```python
from build123d import *

# Parameters (mm, degrees)
F1_DEPTH = 6.35
F2_R     = 10.668
F3_DEPTH = 2.54
F4_DEPTH = 0.254
F6_SIZE2 = 7.62
F6_SIZE  = 1.524
F7_R     = 1.27


with BuildPart() as f1:
    # F0 (on Top) → F1 (new body)
    with BuildSketch(Plane.XY):
        with BuildLine():
            Line((6.711802813, 0.508), (7.7303263191, 0.508))
            ThreePointArc((7.7303263191, 0.508), (5.4779562339, 5.4779562339), (0.508, 7.7303263191))
            Line((0.508, 7.7303263191), (0.508, 6.711802813))
            ThreePointArc((0.508, 6.711802813), (4.7595357442, 4.7595357442), (6.711802813, 0.508))
        make_face()
    extrude(amount=F1_DEPTH)


with BuildPart() as f1b:
    # F0 (on Top) → F1, piece 2 (new body)
    with BuildSketch(Plane.XY):
        with BuildLine():
            ThreePointArc((-0.508, 7.7303263191), (-5.4779562339, 5.4779562339), (-7.7303263191, 0.508))
            Line((-7.7303263191, 0.508), (-6.711802813, 0.508))
            ThreePointArc((-6.711802813, 0.508), (-4.7595357442, 4.7595357442), (-0.508, 6.711802813))
            Line((-0.508, 6.711802813), (-0.508, 7.7303263191))
        make_face()
    extrude(amount=F1_DEPTH)


with BuildPart() as f1c:
    # F0 (on Top) → F1, piece 3 (new body)
    with BuildSketch(Plane.XY):
        with BuildLine():
            Line((-6.711802813, -0.508), (-7.7303263191, -0.508))
            ThreePointArc((-7.7303263191, -0.508), (-5.4779562339, -5.4779562339), (-0.508, -7.7303263191))
            Line((-0.508, -7.7303263191), (-0.508, -6.711802813))
            ThreePointArc((-0.508, -6.711802813), (-4.7595357442, -4.7595357442), (-6.711802813, -0.508))
        make_face()
    extrude(amount=F1_DEPTH)


with BuildPart() as f1d:
    # F0 (on Top) → F1, piece 4 (new body)
    with BuildSketch(Plane.XY):
        with BuildLine():
            ThreePointArc((0.508, -7.7303263191), (5.4779562339, -5.4779562339), (7.7303263191, -0.508))
            Line((7.7303263191, -0.508), (6.711802813, -0.508))
            ThreePointArc((6.711802813, -0.508), (4.7595357442, -4.7595357442), (0.508, -6.711802813))
            Line((0.508, -6.711802813), (0.508, -7.7303263191))
        make_face()
    extrude(amount=F1_DEPTH)


with BuildPart() as f3:
    # F2 (on Top) → F3 (new body)
    with BuildSketch(Plane.XY):
        Circle(F2_R)
    extrude(amount=-F3_DEPTH)


with BuildPart() as f4:
    # F4 (new): a face of the model
    f4_faces = [f3.part.faces().sort_by_distance(p)[0] for p in [
        (0, 0, 0),
    ]]
    extrude(f4_faces, amount=F4_DEPTH)


with BuildPart() as f1c_1:
    add(f1c.part)

    # F5: union F1b, F1, F1d, F3, F4
    add(f1b.part)
    add(f1.part)
    add(f1d.part)
    add(f3.part)
    add(f4.part)

    # F6
    f6_edges = [f1c_1.edges().sort_by_distance(p)[0] for p in [
        (-10.668, 0, -2.54),
    ]]
    f6_side = f1c_1.faces().sort_by_distance((-10.668, 0, -1.143))[0]
    chamfer(f6_edges, length=F6_SIZE, length2=F6_SIZE2, reference=f6_side)

    # F7
    f7_edges = [f1c_1.edges().sort_by_distance(p)[0] for p in [
        (-10.668, 0, -1.016),
        (-3.048, 0, -2.54),
    ]]
    fillet(f7_edges, radius=F7_R)


solid = f1c_1.part
```
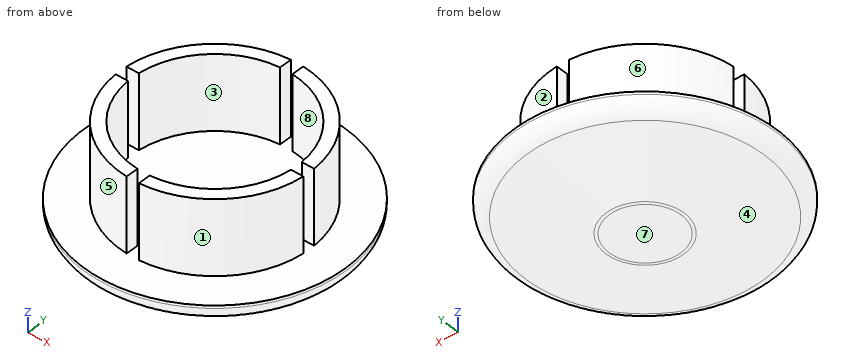
Work out the finished part from the listing and answer in its coordinate system (mm). Face numbers are marked on the shaded views. A direction names the side the tool comes from. Give positions to 0.01 mm unless a question says otherwise; leave off trailing zeros. Loops run counter-clockwise (first coordinate to the right, second up) from the corner with the lowest first, then second, coordinate; pieces in that order, holes last. Notation, with made-up numbers: (-30.5, 28.5) - (24.5, 28.5) arc R25 cw to (24.5, 62.5) - close; hole circle Ø2 at (35.5, 11). An arc over 180 degrees is marked (long way). Use CSV: the item, a comma, the result in double quotes. Start each with the question number.
(1) A tool of negligible diameter and unlimited length cuts with its end or side. For the marked faces 1, 2, 3, 4 and 5, from which of +Z, -Z, +X, -X, +Y, -Y can it reach the whole face along a straight path? Write none if from no direction.
(2) Find section A-A, the plane z = 2.75. Determine the outline of the cut face in (x, y), plus the area to 3 significant figures.
(3) Find the intervals of material crossed by L1, parallel to Z at x = 1.75, y = 2; L2, parallel to Y at x = -3, z = 1.25; L3, parallel to Y at x = -2.25, z = 2, in increasing order.
(4) Each of these flat-tipped pins is pushed along its axis until it touches: pin 1 (6 mm diameter, centred on x = -4.5, y = 5, fed in from -Z); pin 2 (1 mm diameter, centred on x = -3.5, y = -2, fed in from +Z); pin 3 (0.5 mm diameter, centred on y = -7, z = 2, fed in from +X). Where does it stop, or does it pass through?
(5) Determine the mould class of the marked faces 6, 7 and 8 for opening direction Y: released by +Y, released by -Y, zero draft, split by the parting line, or undercut.
Results found:
1,face 1,"+Z, +X, -Y"
1,face 2,"+Z, +X, +Y"
1,face 3,"+Z"
1,face 4,"-Z"
1,face 5,"+Z, -X, -Y"
2,outline,"(-7.73, -0.51) arc R7.75 ccw to (-0.51, -7.73) - (-0.51, -6.71) arc R6.73 cw to (-6.71, -0.51) - close; (-7.73, 0.51) - (-6.71, 0.51) arc R6.73 cw to (-0.51, 6.71) - (-0.51, 7.73) arc R7.75 ccw to start; (0.51, -7.73) arc R7.75 ccw to (7.73, -0.51) - (6.71, -0.51) arc R6.73 cw to (0.51, -6.71) - close; (0.51, 6.71) arc R6.73 cw to (6.71, 0.51) - (7.73, 0.51) arc R7.75 ccw to (0.51, 7.73) - close"
2,area,"42.1 mm^2"
3,L1,"-2.54 to 0.25"
3,L2,"-7.14 to -6.03, 6.03 to 7.14"
3,L3,"-7.41 to -6.34, 6.34 to 7.41"
4,pin 1,"z = -2.4"
4,pin 2,"z = 0.25"
4,pin 3,"x = 3.8"
5,face 6,"released by +Y"
5,face 7,"zero draft"
5,face 8,"undercut"
